The model under review builds one solid part; all positions refer to its coordinate system, in mm. A direction names the side the tool comes from. Round coordinates to 2 decimals unless told otherwise and drop trailing zeros. Order: outer loops, then holes, each group sorted by start corner. A loop starts at its lowest first (then second) coordinate and runs counter-clockwise, first axis right, second up.
1) Consider section A-A (x = 12). Give the boundary of the cut face in (y, z), then the cut area to 3 significant figures.
2) Consider section C-C (z = -4). Give the boundary of the cut face in (x, y).
3) Clearance check with flat-ended pins moving along their axes: P1, Ø2.5, axis at x = 13.5, z = -12, coming from the +Y side; P2, Ø10, axis at y = 20, z = 8, coming from the -X side; P3, Ø17.5, axis at x = -37, z = -20.5, coming from the +Y side. State where each tip first meets the part, or that it passes through.
4) Consider section B-B (y = 37). Give the boundary of the cut face in (x, z), then the cut area to 3 significant figures.
5) Machinability: for faces 5 (the face through (-62.34, 51.197, -16.892)), 6 (the face through (-62.34, 12.16, -10.61)), 7 (the face through (14, 26.818, -18)), 8 (the face through (13.97, 33.77, 12.19)), 9 (the face through (-56.538, -4.039, -17.514)), which of the approach directions +Z, -Z, +X, -X, +Y, -Y give a long, thin tool a straight path to every point of the face, cutting with its end or side? Answer none if there is none.
6) Consider section D-D (y = 10). Give the boundary of the cut face in (x, z).
7) Mouldability with a two-part tool opening along X and no side actions: class faces 1 (the face through (13.97, 34.086, -46.734)), 2 (the face through (-58.348, 26, -18)), 3 (the face through (-66.222, 19, -10)), 4 (the face through (17.852, 19, -17)) as pulls with the +X half, pulls with the -X half, needs draft (parallel to the pull), parting line crosses it, or undercut.
8) To check wall thickness, follow L1, parallel to X at y = 43, z = -19; L2, parallel to Y at x = -62, z = -18.5; L3, parallel to X at y = 40, z = 17.5. State the ranges of each line that lie inside material, in increasing order.
from build123d import *

# Parameters (mm, degrees)
BOSS_EXTRUDE1_DEPTH = 34.544
SKETCH2_R           = 7.112
CUT_EXTRUDE1_DEPTH  = 7.874
BOSS_EXTRUDE2_DEPTH = 7.874
BOSS_EXTRUDE3_DEPTH = 7.874
SKETCH3_3_W         = 34.544
SKETCH3_3_H         = 7.112
CUT_EXTRUDE2_DEPTH  = 34.544
FILLET1_R           = 6.35


with BuildPart() as part:
    # Sketch1 → Boss-Extrude1 (new body)
    with BuildSketch(Plane.XY):
        Polygon((-66.222358974, 33.929598007), (-58.348358974, 33.929598007), (-58.348358974, -5.948401993), (9.977641026, -5.948401993), (9.977641026, 33.929598007), (17.851641026, 33.929598007), (17.851641026, -13.822401993), (-66.222358974, -13.822401993), align=None)
    extrude(amount=-BOSS_EXTRUDE1_DEPTH)

    # Sketch2 → Cut-Extrude1 (cut)
    with BuildSketch(Plane.ZY.offset(66.222358974)):
        with Locations((-17.272, 33.929598007)):
            Circle(SKETCH2_R)
        with Locations((-17.181485908, 14.879598007)):
            Circle(SKETCH2_R)
    extrude(amount=-CUT_EXTRUDE1_DEPTH, mode=Mode.SUBTRACT)

    # Sketch2<3> → Boss-Extrude2 (add)
    with BuildSketch(Plane.ZY.offset(66.222358974)):
        with BuildLine():
            Line((-10.16, 33.929598007), (0, 33.929598007))
            ThreePointArc((0, 33.929598007), (-17.272, 51.201598007), (-34.544, 33.929598007))
            Line((-34.544, 33.929598007), (-24.384, 33.929598007))
            ThreePointArc((-24.384, 33.929598007), (-17.272, 41.041598007), (-10.16, 33.929598007))
        make_face()
    extrude(amount=-BOSS_EXTRUDE2_DEPTH)

    # Sketch3 → Boss-Extrude3 (add)
    with BuildSketch(Plane(origin=(17.851641026, 0, 0), x_dir=(0, 0, -1), z_dir=(1, 0, 0))):
        with BuildLine():
            ThreePointArc((-5.08, 16.93495131), (-5.176663199, 16.935226216), (-5.27332327, 16.936050924))
            ThreePointArc((-5.27332327, 16.936050924), (-1.540900629, 15.352589798), (0, 11.602396048))
            Line((0, 11.602396048), (0, 16.93495131))
            Line((0, 16.93495131), (-5.08, 16.93495131))
        make_face()
        with BuildLine():
            Line((39.624, 50.924244704), (-5.08, 50.924244704))
            ThreePointArc((-5.08, 50.924244704), (-22.074371791, 34.026261206), (-5.27332327, 16.936050924))
            ThreePointArc((-5.27332327, 16.936050924), (-5.176663199, 16.935226216), (-5.08, 16.93495131))
            Line((-5.08, 16.93495131), (0, 16.93495131))
            Line((0, 16.93495131), (0, 26.817598007))
            Line((0, 26.817598007), (-5.08, 26.817598007))
            ThreePointArc((-5.08, 26.817598007), (-12.192, 33.929598007), (-5.08, 41.041598007))
            Line((-5.08, 41.041598007), (39.624, 41.041598007))
            ThreePointArc((39.624, 41.041598007), (46.736, 33.929598007), (39.624, 26.817598007))
            Line((39.624, 26.817598007), (34.544, 26.817598007))
            Line((34.544, 26.817598007), (34.544, 16.93495131))
            Line((34.544, 16.93495131), (39.624, 16.93495131))
            ThreePointArc((39.624, 16.93495131), (39.72066289, 16.935226214), (39.817322653, 16.936050917))
            ThreePointArc((39.817322653, 16.936050917), (56.618371793, 34.026260897), (39.624, 50.924244704))
        make_face()
        with BuildLine():
            ThreePointArc((34.544, 11.602396048), (36.084900412, 15.352589578), (39.817322653, 16.936050917))
            ThreePointArc((39.817322653, 16.936050917), (39.72066289, 16.935226214), (39.624, 16.93495131))
            Line((39.624, 16.93495131), (34.544, 16.93495131))
            Line((34.544, 16.93495131), (34.544, 11.602396048))
        make_face()
    extrude(amount=-BOSS_EXTRUDE3_DEPTH)

    # Sketch3<3> → Cut-Extrude2 (cut)
    with BuildSketch(Plane(origin=(17.851641026, 0, 0), x_dir=(0, 0, -1), z_dir=(1, 0, 0))):
        with Locations((17.272, 30.373598007)):
            Rectangle(SKETCH3_3_W, SKETCH3_3_H)
    extrude(amount=-CUT_EXTRUDE2_DEPTH, mode=Mode.SUBTRACT)

    # Fillet1
    fillet1_edges = [part.edges().sort_by_distance(p)[0] for p in [
        (-58.348358974, -5.948401993, -17.272),
        (9.977641026, -5.948401993, -17.272),
    ]]
    fillet(fillet1_edges, radius=FILLET1_R)


solid = part.part
Answer below:
1. outline: (-13.82, -34.54) - (11.6, -34.54) arc R5.33 cw to (16.94, -39.82) arc R16.99 ccw to (50.92, -39.62) - (50.92, 5.08) arc R16.99 ccw to (16.94, 5.27) arc R5.33 cw to (11.6, 0) - (-13.82, 0) - close; hole (26.82, -39.62) arc R7.11 ccw to (41.04, -39.62) - (41.04, 5.08) arc R7.11 ccw to (26.82, 5.08) - close
1. area: 2,710 mm2
2. outline: (-66.22, -13.82) - (17.85, -13.82) - (17.85, 26.82) - (9.98, 26.82) - (9.98, 0.4) arc R6.35 cw to (3.63, -5.95) - (-52, -5.95) arc R6.35 cw to (-58.35, 0.4) - (-58.35, 44.98) - (-66.22, 44.98) - close; (9.98, 41.04) - (17.85, 41.04) - (17.85, 50.92) - (9.98, 50.92) - close
3. P1: stops at y = 50.92
3. P2: stops at x = 9.98
3. P3: stops at y = -5.95
4. outline: (-66.22, -34.27) - (-58.35, -34.27) - (-58.35, -23.69) - (-66.22, -23.69) - close; (-66.22, -10.86) - (-58.35, -10.86) - (-58.35, -0.28) - (-66.22, -0.28) - close; (9.98, -56.34) - (17.85, -56.34) - (17.85, -46.04) - (9.98, -46.04) - close; (9.98, 11.5) - (17.85, 11.5) - (17.85, 21.79) - (9.98, 21.79) - close
4. area: 329 mm2
5. face 5: -X, +Y
5. face 6: -X
5. face 7: +X
5. face 8: +X, -X
5. face 9: +Z, -Z, +Y
6. outline: (-66.22, -34.54) - (-58.35, -34.54) - (-58.35, -22.36) - (-66.22, -22.36) - close; (-66.22, -12.01) - (-58.35, -12.01) - (-58.35, 0) - (-66.22, 0) - close; (9.98, -34.54) - (17.85, -34.54) - (17.85, 0) - (9.98, 0) - close
7. face 1: needs draft
7. face 2: undercut
7. face 3: pulls with the -X half
7. face 4: pulls with the +X half
8. L1: x = -66.22 to -58.35, 9.98 to 17.85
8. L2: y = -13.82 to 7.89, 21.87 to 26.92, 40.93 to 51.16
8. L3: x = 9.98 to 17.85
